Build history of the part. All positions in model axes, mm. Coordinates: 2 decimals unless noted, no trailing zeros. Order: outer loops, then holes, each group sorted by start corner. A loop starts at its lowest first (then second) coordinate and runs counter-clockwise, first axis right, second up. Notation, with made-up numbers: M 31,8 L 56,8 A22 cw 56,32 Z; hole C -2.75,-8.5 d8. An arc over 180 degrees is marked long. Use a Markdown table: item, result. Add a question column.
from build123d import *

# Parameters (mm, degrees)
SKETCH2_R           = 1.6
SKETCH2_R_2         = 1.5
BOSS_EXTRUDE2_DEPTH = 5
FILLET1_R           = 3


with BuildPart() as part:
    # Sketch2 → Boss-Extrude2 (new body)
    with BuildSketch(Plane(origin=(0, 0, 0), x_dir=(1, 0, 0), z_dir=(0, 1, 0))):
        Polygon((12.701705922, -28), (43.672062905, -28), (-9.649224004, 10.712946228), align=None)
        Circle(SKETCH2_R, mode=Mode.SUBTRACT)
        with Locations((14.43375673, -25)):
            Circle(SKETCH2_R_2, mode=Mode.SUBTRACT)
        with Locations((34.43375673, -25)):
            Circle(SKETCH2_R_2, mode=Mode.SUBTRACT)
    extrude(amount=BOSS_EXTRUDE2_DEPTH)

    # Fillet1
    fillet1_edges = [part.edges().sort_by_distance(p)[0] for p in [
        (43.672062905, 2.5, 28),
        (12.701705922, 2.5, 28),
        (-9.649224004, 2.5, -10.712946228),
    ]]
    fillet(fillet1_edges, radius=FILLET1_R)


solid = part.part
(1) Drop flat-ended pins along their axis: P1, Ø3, axis at y = 1.5, z = 3.5, coming from the +X side; P2, Ø1, axis at x = 30, y = 3.5, coming from the -Z side; P3, Ø1.8, axis at x = 34.43, z = 25, coming from the -Y side; P4, Ø1, axis at y = 4.5, z = 17.5, coming from the -X side. Give the stop position or say it passes through.
(2) Slice it at A-A on y = 3. Give the cut face in (x, z).
(3) Drill centre lines: line 1 along X through (y, z) = (3.7, 25); line 2 along X through (y, z) = (0.6, 26); line 3 along Z through (x, y) = (-1, 3.45). Where is each one in solid material? Low to high. Write a range as from..to.
(4) Mould opens along X. For faces 1 (the cylindrical face through (14.238, 2.465, 23.513)), 2 (the cylindrical face through (-2.05, 2.54, -2.19)), 3 (the flat face through (17, 5, 16)), 4 (the cylindrical face through (33.328, 2.465, 23.986)) say: released by +X, released by -X, zero draft, split by the parting line, or undercut.
(5) Slice it at C-C on z = 25. Give the cut face in (x, y), and give its area (3 significant figures).
(6) Slice it at D-D on z = 0. Give the cut face in (x, y).
(7) Slice it at B-B on x = 0. Give the cut face in (y, z), and give its area (3 significant figures).
Solutions:
| question | item | result |
|---|---|---|
| 1 | P1 | x = 11.99 |
| 1 | P2 | z = 17.71 |
| 1 | P3 | through |
| 1 | P4 | x = 6.35 |
| 2 | outline | M -2.6,1.5 A3 ccw 1.76,-2.43 L 36.2,22.57 A3 ccw 34.43,28 L 14.43,28 A3 ccw 11.84,26.5 Z; hole C 0,0 d3.2; hole C 14.43,25 d3; hole C 34.43,25 d3 |
| 3 | line 1 | 10.97..12.93, 15.93..32.93, 35.93..37.43 |
| 3 | line 2 | 11.55..13.32, 15.55..33.32, 35.55..37.26 |
| 3 | line 3 | -2.83..-1.25, 1.25..4.27 |
| 4 | face 1 | undercut |
| 4 | face 2 | split by the parting line |
| 4 | face 3 | zero draft |
| 4 | face 4 | undercut |
| 5 | outline | M 10.97,0 L 12.93,0 L 12.93,5 L 10.97,5 Z; M 15.93,0 L 32.93,0 L 32.93,5 L 15.93,5 Z; M 35.93,0 L 37.43,0 L 37.43,5 L 35.93,5 Z |
| 5 | area | 102 mm² |
| 6 | outline | M -3,0 L -1.6,0 L -1.6,5 L -3,5 Z; M 1.6,0 L 5.11,0 L 5.11,5 L 1.6,5 Z |
| 7 | outline | M 0,-3 L 5,-3 L 5,-1.6 L 0,-1.6 Z; M 0,1.6 L 5,1.6 L 5,6 L 0,6 Z |
| 7 | area | 29.0 mm² |
